```python
from build123d import *

# Parameters (mm, degrees)
BOSS_EXTRUDE1_DEPTH = 1.5875


with BuildPart() as part:
    # Sketch1 → Boss-Extrude1 (new body)
    with BuildSketch(Plane(origin=(0, 0, 0), x_dir=(1, 0, 0), z_dir=(0, 1, 0))):
        with BuildLine():
            Line((0, 90), (100, 90))
            Line((100, 90), (100, 0))
            Line((100, 0), (93.75, 0))
            Line((93.75, 0), (93.75, 4.625))
            Line((93.75, 4.625), (90.25, 4.625))
            Line((90.25, 4.625), (90.25, 0))
            Line((90.25, 0), (84, 0))
            ThreePointArc((84, 0), (81.178095625, 1.089694192), (79.99799, 3.875))
            Line((79.99799, 3.875), (80, 4))
            Line((80, 4), (80, 7))
            Line((80, 7), (80.00201, 7.125))
            ThreePointArc((80.00201, 7.125), (78.821904375, 9.910305808), (76, 11))
            Line((76, 11), (53.25, 11))
            ThreePointArc((53.25, 11), (50.428095625, 9.910305808), (49.24799, 7.125))
            Line((49.24799, 7.125), (49.25, 7))
            Line((49.25, 7), (49.25, 4))
            Line((49.25, 4), (49.25201, 3.87502))
            ThreePointArc((49.25201, 3.87502), (48.071906674, 1.089706193), (45.25, 0))
            Line((45.25, 0), (43.75, 0))
            Line((43.75, 0), (43.75, 4.625))
            Line((43.75, 4.625), (40.25, 4.625))
            Line((40.25, 4.625), (40.25, 0))
            Line((40.25, 0), (35.75, 0))
            Line((35.75, 0), (35.75, 4.625))
            Line((35.75, 4.625), (32.25, 4.625))
            Line((32.25, 4.625), (32.25, 0))
            Line((32.25, 0), (26.75, 0))
            Line((26.75, 0), (26.75, 4.625))
            Line((26.75, 4.625), (23.25, 4.625))
            Line((23.25, 4.625), (23.25, 0))
            Line((23.25, 0), (17.75, 0))
            Line((17.75, 0), (17.75, 4.625))
            Line((17.75, 4.625), (14.25, 4.625))
            Line((14.25, 4.625), (14.25, 0))
            Line((14.25, 0), (8.75, 0))
            Line((8.75, 0), (8.75, 4.625))
            Line((8.75, 4.625), (5.25, 4.625))
            Line((5.25, 4.625), (5.25, 0))
            Line((5.25, 0), (0, 0))
            Line((0, 0), (0, 90))
        make_face()
    extrude(amount=BOSS_EXTRUDE1_DEPTH)


solid = part.part
```
Here's how the part is built. I have some questions about the finished solid (model axes, mm). A direction names the side the tool comes from. Coordinates: 2 decimals unless noted, no trailing zeros.
1) Will these pins go through, and if not, where does the flat tip stop? pin 1 (0.5 mm diameter, centred on x = 29.5, y = 1, fed in from +Z); pin 2 (0.5 mm diameter, centred on x = 15, y = 1, fed in from +Z) (3 decimals).
2) Which directions (+Z, -Z, +X, -X, +Y, -Y) give clear straight access to the entire face, cutting with the end or side of a thin tool? Please do faces 1 (the face through (48.103, 0.783, -1.12)), 2 (the face through (51, 0, -46)).
3) I need wall thicknesses on line 1 (Z direction, x = 31.5, y = 0.3); line 2 (Z direction, x = 65, y = 0.1). Which ranges of each line are inside material? Lowest first, please.
4) We'd pull the mould along X, two halves only. Please class faces 3 (the face through (81.21, 0.78, -1.06)), 4 (the face through (51, 1.588, -46)): +X half, -X half, draft (parallel to the pull), parting line (faces both ways), or undercut.
Response values:
1. pin 1: stops at z = 0
1. pin 2: stops at z = -4.625
2. face 1: +Z, +Y, -Y
2. face 2: +Z, -Z, +X, -X, -Y
3. line 1: z = -90 to 0
3. line 2: z = -90 to -11
4. face 3: undercut
4. face 4: draft
